Check sheet for the modelled part. Datum: model origin and axes. Units: mm. A direction names the side the tool comes from. Give positions to 0.01 mm unless a question says otherwise; leave off trailing zeros. Order: outer loops, then holes, each group sorted by start corner. A loop starts at its lowest first (then second) coordinate and runs counter-clockwise, first axis right, second up. Notation, with made-up numbers: (-24, 3) -> (-17, 3) arc R12 ccw to (-17, 11) -> close; hole circle Ø1 at (3, 38). An arc over 180 degrees is marked (long way). One line per question, with ' | ' between items.
Autodesk Inventor part; units mm, degrees
ref_plane "YZ Plane" through (0, 0, 0) normal (1, 0, 0) x (0, 1, 0)
ref_plane "XZ Plane" through (0, 0, 0) normal (0, 1, 0) x (-1, 0, 0)
ref_plane "XY Plane" through (0, 0, 0) normal (0, 0, 1) x (1, 0, 0)
sketch "Sketch1" plane through (0, 0, 0) normal (0, 1, 0) x (-1, 0, 0)
  line L0 (-4.7625, -17.4625) -> (4.7625, -17.4625)
  line L1 (4.7625, -17.4625) -> (4.7625, 17.4625)
  line L2 (4.7625, 17.4625) -> (-4.7625, 17.4625)
  line L3 (-4.7625, -17.4625) -> (4.7625, 17.4625) construction
  line L4 (4.7625, -17.4625) -> (-4.7625, 17.4625) construction
  line L5 (1.5875, -12.7) -> (1.5875, 12.7)
  line L6 (1.5875, 12.7) -> (-11.1125, -12.7) construction
  line L7 (-11.1125, 12.7) -> (1.5875, -12.7) construction
  line L8 (1.5875, 12.7) -> (-4.7625, 12.7)
  line L9 (1.5875, -12.7) -> (-4.7625, -12.7)
  line L10 (-4.7625, 12.7) -> (-4.7625, 17.4625)
  line L11 (-4.7625, -12.7) -> (-4.7625, -17.4625)
  point P0 (0, 0)
  point P1 (-4.7625, 0)
  dimension "d0" = 9.525
  dimension "d1" = 34.925
  dimension "d2" = 12.7
  dimension "d3" = 25.4
extrude "Extrusion1" add sketch "Sketch1" along normal blind 304.8
properties part number "14in-slide-pt_2" material "Aluminum 6061"
Q1. Mould release check, pull along Z, two halves, no side actions. Record for faces 3 (the face through (2, 150, 12.7)), 4 (the face through (0, 150, -17.462)), 5 (the face through (-2, 304.8, 0)), 6 (the face through (0, 150, 17.462)): pulls with the +Z half, pulls with the -Z half, needs draft (parallel to the pull), parting line crosses it, or undercut.
Result sheet:
face 3: undercut | face 4: pulls with the -Z half | face 5: needs draft | face 6: pulls with the +Z half
Q2. Depth check by flat-ended pin: pin 1 Ø12.5 at (y, z) = (105.5, -2.5) entering from +X. Enter the tip coordinate at first touch or a pass-through.
Result sheet:
pin 1: stops at x = -1.59
Q3. Access from +Z, -Z, +X, -X, +Y, -Y to the whole of each face (thin tool, end or side, straight path). Record for faces 1 (the face through (-4.762, 150, 0)), 2 (the face through (2, 150, -12.7)).
Result sheet:
face 1: +Z, -Z, -X, +Y, -Y | face 2: +X, +Y, -Y
Q4. Section check A-A (x = 0.25). Enter the section's corners in (y, z).
Result sheet:
outline: (0, -17.46) -> (304.8, -17.46) -> (304.8, -12.7) -> (0, -12.7) -> close; (0, 12.7) -> (304.8, 12.7) -> (304.8, 17.46) -> (0, 17.46) -> close
Q5. Thickness scan on line 1 (Z direction, x = 0.75, y = 196); line 2 (X direction, y = 102.5, z = -4.5). Record the ranges inside material, lowest first.
Result sheet:
line 1: z = -17.46 to -12.7, 12.7 to 17.46 | line 2: x = -4.76 to -1.59
Q6. Section check C-C (z = 8). Enter the section's corners in (x, y), and give its area (3 significant figures).
Result sheet:
outline: (-4.76, 0) -> (-1.59, 0) -> (-1.59, 304.8) -> (-4.76, 304.8) -> close | area: 968 mm2
Q7. Section check B-B (y = 87). Enter the section's corners in (x, z), and give its area (3 significant figures).
Result sheet:
outline: (-4.76, -17.46) -> (4.76, -17.46) -> (4.76, -12.7) -> (-1.59, -12.7) -> (-1.59, 12.7) -> (4.76, 12.7) -> (4.76, 17.46) -> (-4.76, 17.46) -> close | area: 171 mm2
